```python
from build123d import *

# Parameters (mm, degrees)
F2_W     = 1.7657947028
F2_H     = 4.3581165373
F4_DEPTH = 6.35
F5_W     = 0.7065157406
F5_H     = 3.5888564307
F7_DEPTH = 13.97


with BuildPart() as f1:
    # F0 (on Front) → F1 (revolve)
    with BuildSketch(Plane.XZ):
        Polygon((0, 33.02), (0, 0), (8.1676599603, 14.0551366686), (18.0931817596, 19.7233742263), (8.1676599603, 25.391611784), (4.0838299801, 29.205805892), align=None)
        Polygon((4.0838299801, 33.5109336315), (0, 33.02), (4.0838299801, 29.205805892), align=None)
    revolve(axis=Axis((0, 0, 16.51), (0, 0, -1)))

    # F2 (on Front) → F3 (revolve)
    with BuildSketch(Plane.XZ):
        with Locations((0.8828973514, 31.3695054501)):
            Rectangle(F2_W, F2_H)
    revolve(axis=Axis((0, 0, 31.3695054501), (0, 0, 1)))

    # F4 (cut, symmetric): a face of the model
    f4_faces = [f1.faces().sort_by_distance(p)[0] for p in [
        (0, 0, 33.5485637188),
    ]]
    extrude(f4_faces, amount=F4_DEPTH, both=True, mode=Mode.SUBTRACT)

    # F5 (on Front) → F6 (revolve)
    with BuildSketch(Plane.XZ):
        with Locations((0.3532578703, 1.7944282154)):
            Rectangle(F5_W, F5_H)
    revolve(axis=Axis((0, 0, 1.7944282154), (0, 0, -1)))

    # F7 (cut): a face of the model
    f7_faces = [f1.faces().sort_by_distance(p)[0] for p in [
        (0, 0, 0),
    ]]
    extrude(f7_faces, amount=-F7_DEPTH, mode=Mode.SUBTRACT)


solid = f1.part
```
Build history of the part. All positions in model axes, mm. A direction names the side the tool comes from. Coordinates: 2 decimals unless noted, no trailing zeros. Write each loop counter-clockwise with the first axis right and the second up, starting at its lowest first coordinate (ties: lowest second). Pieces come first, ordered by that corner, then holes.
1. Drop flat-ended pins along their axis: pin 1 (3 mm diameter, centred on x = 0, y = 0, fed in from +Z); pin 2 (3 mm diameter, centred on x = 8.5, y = -3.5, fed in from +Z); pin 3 (1.5 mm diameter, centred on x = 11.5, y = -11, fed in from +Z). Give the stop position or say it passes through.
Answer block:
pin 1: stops at z = 27.2
pin 2: stops at z = 25.84
pin 3: stops at z = 21.4
2. Band-saw the part on C-C, the plane z = 11. Give the cut face in (x, y).
Answer block:
outline: circle Ø12.78 at (0, 0); hole circle Ø1.41 at (0, 0)
3. Band-saw the part on A-A, the plane y = 0. Give the cut face in (x, z).
Answer block:
outline: (-18.09, 19.72) - (-8.17, 14.06) - (-0.71, 1.22) - (-0.71, 13.97) - (0.71, 13.97) - (0.71, 1.22) - (8.17, 14.06) - (18.09, 19.72) - (8.17, 25.39) - (4.08, 29.21) - (4.08, 33.51) - (1.77, 33.23) - (1.77, 27.2) - (-1.77, 27.2) - (-1.77, 33.23) - (-4.08, 33.51) - (-4.08, 29.21) - (-8.17, 25.39) - close
4. Drill centre lines: probe 1 along Y at (x, z) = (0, 29.25); probe 2 along X at (y, z) = (0, 4); probe 3 along Y at (x, z) = (0, 11). Where is each one in solid material? Low to high.
Answer block:
probe 1: y = -4.08 to -1.77, 1.77 to 4.08
probe 2: x = -2.32 to -0.71, 0.71 to 2.32
probe 3: y = -6.39 to -0.71, 0.71 to 6.39
5. 3-axis set-ups, long thin cutter, end or side, ignore diameter. For faces 1 (the cylindrical face through (-0.15, 0.69, 7.5)), 2 (the flat face through (0, 0, 27.199)): which of +Z, -Z, +X, -X, +Y, -Y reach the whole face in a straight line?
Answer block:
face 1: -Z
face 2: +Z
6. Band-saw the part on D-D, the plane z = 26. Give the cut face in (x, y).
Answer block:
outline: circle Ø15.03 at (0, 0)
7. Pull direction X, two halves, no side cores. Call faces 3 (the conical face through (1.69, 3.25, 6.3)), 4 (the flat face through (0, 0, 13.97)), 5 (the cylindrical face through (-0.383, -1.724, 30.258)): released by +X, released by -X, zero draft, split by the parting line, or undercut.
Answer block:
face 3: split by the parting line
face 4: undercut
face 5: undercut
